```python
from build123d import *

# Parameters (mm, degrees)
SZKIC1_W                = 60
SZKIC1_H                = 60
SZKIC1_R                = 21
ODGI_CIE_BAZOWE1_DEPTH  = 4
OTW_R_POD_RUB_M51_D     = 5.5
OTW_R_POD_RUB_M51_DEPTH = 11
OTW_R_POD_RUB_M51_TIP   = 1.652366702
SFAZOWANIE1_SIZE        = 3


# Sheet-metal steps are written as plain solids
with BuildPart() as part:
    # Szkic1 → Odgięcie bazowe1 (new body)
    with BuildSketch(Plane(origin=(0, 0, 0), x_dir=(0, 0, -1), z_dir=(1, 0, 0))):
        Rectangle(SZKIC1_W, SZKIC1_H)
        Circle(SZKIC1_R, mode=Mode.SUBTRACT)
    extrude(amount=-ODGI_CIE_BAZOWE1_DEPTH)

    # Otwór pod śrubę M51
    with Locations(Plane(origin=(0, 0, 0), x_dir=(0, 0, -1), z_dir=(1, 0, 0))):
        with Locations((-23.575, 23.575), (23.575, 23.575), (23.575, -23.575), (-23.575, -23.575)):
            Hole(OTW_R_POD_RUB_M51_D / 2, depth=OTW_R_POD_RUB_M51_DEPTH)
            with Locations((0, 0, -(OTW_R_POD_RUB_M51_DEPTH + OTW_R_POD_RUB_M51_TIP / 2))):  # 118° drill point
                Cone(0, OTW_R_POD_RUB_M51_D / 2, OTW_R_POD_RUB_M51_TIP, mode=Mode.SUBTRACT)

    # Sfazowanie1
    sfazowanie1_edges = [part.edges().sort_by_distance(p)[0] for p in [
        (-2, -30, -30),
        (-2, -30, 30),
        (-2, 30, 30),
        (-2, 30, -30),
    ]]
    chamfer(sfazowanie1_edges, length=SFAZOWANIE1_SIZE)


solid = part.part
```
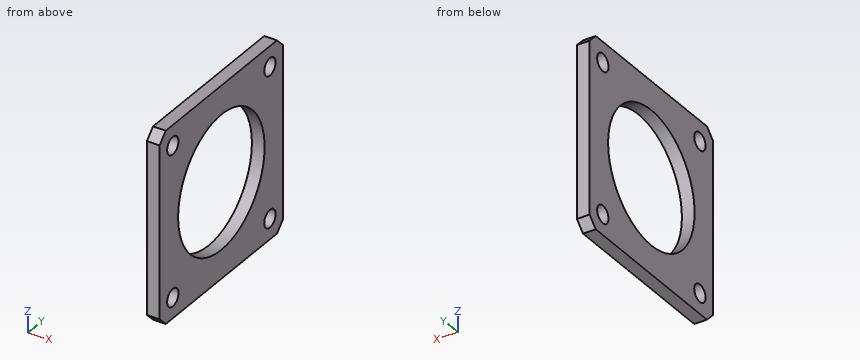
For this review, take the finished solid that the model builds, in its own axes (mm). Coordinates: 2 decimals unless noted, no trailing zeros. Order: outer loops, then holes, each group sorted by start corner. A loop starts at its lowest first (then second) coordinate and runs counter-clockwise, first axis right, second up. Notation, with made-up numbers: (69, 54.25) - (81, 54.25) arc R25 ccw to (81, 89.25) - close; hole circle Ø10 at (3.25, 38). An arc over 180 degrees is marked (long way). Answer as a JSON object with one key per item and string values. Group by question number.
1. We need section A-A on y = 0. State the section outline as (x, z) points.
2. We need section D-D on x = -2.8. State the section outline as (y, z) points (3 decimals).
3. Clearance check with a flat-ended pin moving along its axis: P1, Ø6.5, axis at y = -23.575, z = 23.575, coming from the +X side. State where the tip first meets the part, or that it passes through.
4. We need section C-C on z = 25.5. State the section outline as (x, y) points.
5. For probe 1 along Y at (x, z) = (-2.5, 0); probe 2 along Z at (x, y) = (-0.7, 17.5); probe 3 along Y at (x, z) = (-3.35, 1.5), list the stretches that pass through material, from the lowest coordinate up.
Final values:
{
 "1": {"outline": "(-4, -30) - (0, -30) - (0, -21) - (-4, -21) - close; (-4, 21) - (0, 21) - (0, 30) - (-4, 30) - close"},
 "2": {"outline": "(-30, -27) - (-27, -30) - (27, -30) - (30, -27) - (30, 27) - (27, 30) - (-27, 30) - (-30, 27) - close; hole circle Ø5.5 at (-23.575, -23.575); hole circle Ø5.5 at (-23.575, 23.575); hole circle Ø42 at (0, 0); hole circle Ø5.5 at (23.575, -23.575); hole circle Ø5.5 at (23.575, 23.575)"},
 "3": {"P1": "x = 0"},
 "4": {"outline": "(-4, -30) - (0, -30) - (0, -25.54) - (-4, -25.54) - close; (-4, -21.61) - (0, -21.61) - (0, 21.61) - (-4, 21.61) - close; (-4, 25.54) - (0, 25.54) - (0, 30) - (-4, 30) - close"},
 "5": {"probe 1": "-30 to -21, 21 to 30", "probe 2": "-30 to -11.61, 11.61 to 30", "probe 3": "-30 to -20.95, 20.95 to 30"}
}
